Geometry: final body of the model. Coordinates: model frame, mm. A direction names the side the tool comes from. Coordinates: 2 decimals unless noted, no trailing zeros. Loops run counter-clockwise (first coordinate to the right, second up) from the corner with the lowest first, then second, coordinate; pieces in that order, holes last. Notation, with made-up numbers: (-6, 12) - (26, 12) arc R23 cw to (26, 37) - close; hole circle Ø6 at (72, -19). An arc over 180 degrees is marked (long way). Answer in a Markdown table with one row per item.
from build123d import *

# Parameters (mm, degrees)
BOSS_EXTRUDE1_DEPTH = 4
SKETCH2_W           = 9
SKETCH2_H           = 17.5
SKETCH2_W_2         = 57
SKETCH2_H_2         = 9
BOSS_EXTRUDE2_DEPTH = 1.7
CHAMFER1_SIZE       = 1.7
SKETCH4_R           = 2.625
CUT_EXTRUDE1_DEPTH  = 70.019852217
FILLET1_R           = 1


with BuildPart() as part:
    # Sketch1 → Boss-Extrude1 (new body)
    with BuildSketch(Plane(origin=(0, 0, 0), x_dir=(1, 0, 0), z_dir=(0, 1, 0))):
        Polygon((0, 0), (57, 0), (57, 20), (38.5, 38.5), (18.5, 38.5), (0, 20), align=None)
    extrude(amount=BOSS_EXTRUDE1_DEPTH)

    # Sketch2 → Boss-Extrude2 (add)
    with BuildSketch(Plane(origin=(0, 4, 0), x_dir=(1, 0, 0), z_dir=(0, 1, 0))):
        with Locations((28.5, 29.75)):
            Rectangle(SKETCH2_W, SKETCH2_H)
        with Locations((28.5, 10)):
            Rectangle(SKETCH2_W_2, SKETCH2_H_2)
    extrude(amount=BOSS_EXTRUDE2_DEPTH)

    # Chamfer1
    chamfer1_edges = [part.edges().sort_by_distance(p)[0] for p in [
        (33, 5.7, -29.75),
        (28.5, 5.7, -14.5),
        (24, 5.7, -29.75),
        (28.5, 5.7, -5.5),
    ]]
    chamfer(chamfer1_edges, length=CHAMFER1_SIZE - 0.0001)  # a hair under: the kernel refuses the full size

    # Sketch4 → Cut-Extrude1 (cut, through all)
    with BuildSketch(Plane.XZ):
        with Locations(Location((10, -10, 0), (0, 0, 270))):
            Circle(SKETCH4_R)
        with Locations(Location((47, -10, 0), (0, 0, 270))):
            Circle(SKETCH4_R)
        with Locations(Location((28.5, -28.5, 0), (0, 0, 270))):
            Circle(SKETCH4_R)
    extrude(amount=-CUT_EXTRUDE1_DEPTH, mode=Mode.SUBTRACT)

    # Fillet1
    fillet1_edges = [part.edges().sort_by_distance(p)[0] for p in [
        (0, 2, -20),
        (18.5, 2, -38.5),
        (38.5, 2, -38.5),
        (57, 2, -20),
        (57, 2, 0),
        (0, 2, 0),
    ]]
    fillet(fillet1_edges, radius=FILLET1_R)


solid = part.part
(1) First-contact query: pin 1 Ø7 at (x, z) = (10, -10) entering from -Y; pin 2 Ø2 at (x, y) = (42, 4) entering from -Z; pin 3 Ø4 at (x, z) = (28.5, -28.5) entering from +Y; pin 4 Ø1.5 at (y, z) = (0.5, -25.5) entering from -X. Flat tips, straight axial feed; report the tip coordinate or a pass-through.
Verdict:
| item | result |
|---|---|
| pin 1 | stops at y = 0 |
| pin 2 | stops at z = -36 |
| pin 3 | passes through |
| pin 4 | stops at x = 4.75 |
(2) Cut plane A-A on z = -10. Output: boundary loops of the cut face in (x, y) (3 decimals), then the cut area to 3 significant figures.
Verdict:
| item | result |
|---|---|
| outline | (0, 0) - (7.375, 0) - (7.375, 5.7) - (0, 5.7) - close; (12.625, 0) - (44.375, 0) - (44.375, 5.7) - (12.625, 5.7) - close; (49.625, 0) - (57, 0) - (57, 5.7) - (49.625, 5.7) - close |
| area | 265 mm² |
(3) Access query for faces 1 (the face through (0, 2, -10)), 2 (the face through (32, 5, -30)), 3 (the face through (28, 5, -21)), 4 (the face through (10.115, 2.81, -7.378)), 5 (the face through (25, 5, -30)). Directions: +Z, -Z, +X, -X, +Y, -Y. A direction counts if a zero-diameter tool reaches every point of the face in a straight line with its end or side. Return the directions, or none.
Verdict:
| item | result |
|---|---|
| face 1 | +Z, -Z, -X, +Y, -Y |
| face 2 | -Z, +X, +Y |
| face 3 | +X, -X, +Y |
| face 4 | +Y, -Y |
| face 5 | -Z, -X, +Y |
(4) Cut plane B-B on y = 2.8. Output: boundary loops of the cut face in (x, z) (3 decimals).
Verdict:
| item | result |
|---|---|
| outline | (0, -19.586) arc R1 ccw to (0.293, -20.293) - (18.207, -38.207) arc R1 ccw to (18.914, -38.5) - (38.086, -38.5) arc R1 ccw to (38.793, -38.207) - (56.707, -20.293) arc R1 ccw to (57, -19.586) - (57, -1) arc R1 ccw to (56, 0) - (1, 0) arc R1 ccw to (0, -1) - close; hole circle Ø5.25 at (10, -10); hole circle Ø5.25 at (28.5, -28.5); hole circle Ø5.25 at (47, -10) |
(5) Ray query, probe 1 along X at (y, z) = (1.7, -10) (3 decimals); probe 2 along Y at (x, z) = (48, -16.5); probe 3 along X at (y, z) = (4.1, -28.5) (3 decimals). Return the intervals inside material, ascending.
Verdict:
| item | result |
|---|---|
| probe 1 | x = 0 to 7.375, 12.625 to 44.375, 49.625 to 57 |
| probe 2 | y = 0 to 4 |
| probe 3 | x = 24.1 to 25.875, 31.125 to 32.9 |
(6) Pull-direction query (Z, two-part tool) for faces 6 (the face through (47.115, 2.81, -7.378)), 7 (the face through (28.1, 4.9, -6.4)), 8 (the face through (26.9, 2.81, -26.42)), 9 (the face through (28, 4, -3)); classes: pulls with the +Z half, pulls with the -Z half, needs draft (parallel to the pull), parting line crosses it, or undercut.
Verdict:
| item | result |
|---|---|
| face 6 | undercut |
| face 7 | pulls with the +Z half |
| face 8 | undercut |
| face 9 | needs draft |
